Source: CAD feature listing. Evaluate the final solid. Frame: model axes, mm. A direction names the side the tool comes from. Round coordinates to 2 decimals unless told otherwise and drop trailing zeros. Loops run counter-clockwise (first coordinate to the right, second up) from the corner with the lowest first, then second, coordinate; pieces in that order, holes last. Notation, with made-up numbers: M 40,74 L 85,74 A12 ccw 85,85 Z; hole C 71,-4 d5. An arc over 180 degrees is marked long. One line per item, written item: value.
from build123d import *

# Parameters (mm, degrees)
F1_DEPTH = 40.2336
F0_R     = 10.16
F2_DEPTH = 15.7734
F3_R     = 3.302


with BuildPart() as f1:
    # F0 (on Front) → F1 (new body)
    with BuildSketch(Plane.XZ):
        with BuildLine():
            ThreePointArc((7.395882, -27.601296), (22.670112, -17.395305), (28.575, 0))
            ThreePointArc((28.575, 0), (22.670112, 17.395305), (7.395882, 27.601296))
            ThreePointArc((7.395882, 27.601296), (-28.575, 0), (7.395882, -27.601296))
        make_face()
        with BuildLine():
            ThreePointArc((13.447765, -4.826), (-14.2875, 0), (13.447765, 4.826))
            Line((13.447765, 4.826), (17.689565, 4.826))
            Line((17.689565, 4.826), (17.689565, -4.826))
            Line((17.689565, -4.826), (13.447765, -4.826))
        make_face(mode=Mode.SUBTRACT)
    extrude(amount=F1_DEPTH)

    # F0 (on Front) → F2 (join)
    with BuildSketch(Plane.XZ):
        with BuildLine():
            ThreePointArc((7.395882, 27.601296), (22.670112, 17.395305), (28.575, 0))
            ThreePointArc((28.575, 0), (22.670112, -17.395305), (7.395882, -27.601296))
            Line((7.395882, -27.601296), (57.755118, -14.107329))
            ThreePointArc((57.755118, -14.107329), (39.37, 0), (57.755118, 14.107329))
            Line((57.755118, 14.107329), (7.395882, 27.601296))
        make_face()
        with BuildLine():
            ThreePointArc((68.58, 0), (65.561946, 8.890934), (57.755118, 14.107329))
            ThreePointArc((57.755118, 14.107329), (39.37, 0), (57.755118, -14.107329))
            ThreePointArc((57.755118, -14.107329), (65.561946, -8.890934), (68.58, 0))
        make_face()
        with Locations((53.975, 0)):
            Circle(F0_R, mode=Mode.SUBTRACT)
    extrude(amount=F2_DEPTH)

    # F3
    f3_edges = [f1.edges().sort_by_distance(p)[0] for p in [
        (-7.395882, -40.2336, 27.601296),
    ]]
    fillet(f3_edges, radius=F3_R)


solid = f1.part
1. Pull-direction query (Z, two-part tool) for faces 1 (the face through (32.93, -7.78, 20.76)), 2 (the face through (16, -20, 4.826)), 3 (the face through (11, -40.234, -11)); classes: released by +Z, released by -Z, zero draft, split by the parting line, or undercut.
Report:
face 1: released by +Z
face 2: undercut
face 3: zero draft
2. Section query D-D (x = 33). Return the cut outline in (y, z).
Report:
outline: M -15.77,-20.74 L 0,-20.74 L 0,20.74 L -15.77,20.74 Z
3. Ray query, line 1 (Z direction, x = 0, y = -10) (1 decimal); line 2 (X direction, y = -8.5, z = -5); line 3 (X direction, y = -21.5, z = 0) (1 decimal). Return the intervals inside material, ascending. Write a range as [from, to].
Report:
line 1: z = [-28.6, -14.3], [14.3, 28.6]
line 2: x = [-28.13, -13.38], [13.38, 45.13], [62.82, 67.7]
line 3: x = [-28.6, -14.3], [17.7, 28.6]
4. Reachability of faces 4 (the face through (32.22, -7.78, -20.95)), 5 (the face through (16, -20, -4.826)) from +Z, -Z, +X, -X, +Y, -Y: full face, straight path, thin tool, end or side. Return the list, or none.
Report:
face 4: -Z, +X, +Y, -Y
face 5: +Y, -Y
5. Pin query (flat end, axial travel): pin 1 (7.5 mm diameter, centred on y = -19, z = 2.5, fed in from -X) (3 decimals); pin 2 (1.3 mm diameter, centred on x = 15, y = -20, fed in from +Z); pin 3 (1 mm diameter, centred on y = -31.5, z = 10.5, fed in from -X). Return the tip coordinate at first contact, or that it passes through.
Report:
pin 1: stops at x = -28.575
pin 2: stops at z = 24.71
pin 3: stops at x = -26.77
6. Section query A-A (y = -5.5). Count the separate pieces of the cut face and the enclosed holes in it, and give its area (3 significant figures).
Report:
separate pieces: 1
enclosed holes: 2
area: 3,030 mm2
